Part model, mm, in its own coordinate system. Give positions to 0.01 mm unless a question says otherwise; leave off trailing zeros. Write each loop counter-clockwise with the first axis right and the second up, starting at its lowest first coordinate (ties: lowest second). Pieces come first, ordered by that corner, then holes. Notation, with made-up numbers: M 82,-10.75 L 125,-10.75 A12 ccw 125,11.25 Z; hole C -30,-39 d6. An arc over 180 degrees is marked long. Use a Markdown table: item, result.
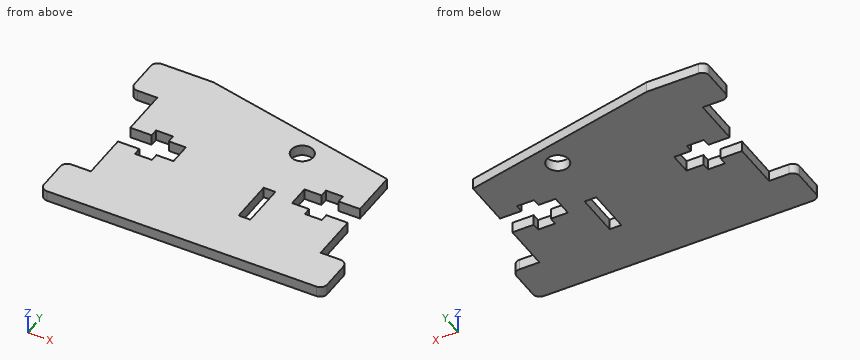
```python
from build123d import *

# Parameters (mm, degrees)
SKETCH_1_R      = 2.05
SKETCH_1_W      = 2.2
SKETCH_1_H      = 8.3
EXTRUDE_1_DEPTH = 2
FILLET_1_R      = 1.3


with BuildPart() as part:
    # 草图1 → 凸台-拉伸1 (new body)
    with BuildSketch(Plane.XY):
        Polygon((-35.523848217, 30.239854129), (-30.523848217, 30.239854129), (12.476151783, 30.239854129), (17.476151783, 30.239854129), (17.476151783, 38.239854129), (12.476151783, 38.239854129), (12.476151783, 47.189854129), (8.476151783, 47.189854129), (8.476151783, 45.739854129), (5.276151783, 45.739854129), (5.276151783, 47.189854129), (2.076151783, 47.189854129), (2.076151783, 51.289854129), (5.276151783, 51.289854129), (5.276151783, 52.739854129), (8.476151783, 52.739854129), (8.476151783, 51.289854129), (12.476151783, 51.289854129), (12.476151783, 60.239854129), (-24.523824953, 68.239854129), (-30.523848217, 68.239854129), (-35.523848217, 68.239854129), (-35.523848217, 60.239854129), (-30.523848217, 60.239854129), (-30.523848217, 51.289854129), (-26.523848217, 51.289854129), (-26.523848217, 52.739854129), (-23.323848217, 52.739854129), (-23.323848217, 51.289854129), (-20.123848217, 51.289854129), (-20.123848217, 47.189854129), (-23.323848217, 47.189854129), (-23.323848217, 45.739854129), (-26.523848217, 45.739854129), (-26.523848217, 47.189854129), (-30.523848217, 47.189854129), (-30.523848217, 38.239854129), (-35.523848217, 38.239854129), align=None)
        with Locations((-2.823848217, 59.239854129)):
            Circle(SKETCH_1_R, mode=Mode.SUBTRACT)
        with Locations((-2.823848217, 44.239854129)):
            Rectangle(SKETCH_1_W, SKETCH_1_H, mode=Mode.SUBTRACT)
    extrude(amount=EXTRUDE_1_DEPTH)

    # 圆角1
    fillet_1_edges = [part.edges().sort_by_distance(p)[0] for p in [
        (-35.523848217, 60.239854129, 1),
        (-35.523848217, 68.239854129, 1),
        (17.476151783, 38.239854129, 1),
        (17.476151783, 30.239854129, 1),
        (-35.523848217, 30.239854129, 1),
        (-35.523848217, 38.239854129, 1),
    ]]
    fillet(fillet_1_edges, radius=FILLET_1_R)


solid = part.part
```
1. Cut at A-A, the plane x = -31.5. Give the cut face in (y, z).
Findings below:
| item | result |
|---|---|
| outline | M 30.24,0 L 38.24,0 L 38.24,2 L 30.24,2 Z; M 60.24,0 L 68.24,0 L 68.24,2 L 60.24,2 Z |
2. Cut at B-B, the plane y = 58. Give the cut face in (x, z).
Findings below:
| item | result |
|---|---|
| outline | M -30.52,0 L -4.46,0 L -4.46,2 L -30.52,2 Z; M -1.19,0 L 12.48,0 L 12.48,2 L -1.19,2 Z |
3. Drop flat-ended pins along their axis: P1, Ø0.6, axis at y = 43, z = 0.5, coming from the -X side; P2, Ø1, axis at y = 38.5, z = 0.5, coming from the +X side; P3, Ø1, axis at x = -2.5, z = 0.5, coming from the +Y side; P4, Ø2, axis at x = 7, y = 45.5, coming from the -Z side. Give the stop position or say it passes through.
Findings below:
| item | result |
|---|---|
| P1 | x = -30.52 |
| P2 | x = 16.93 |
| P3 | y = 63.59 |
| P4 | z = 0 |
4. Drill centre lines: L1, parallel to X at y = 51.5, z = 0.45; L2, parallel to X at y = 46, z = 0.4; L3, parallel to X at y = 40.5, z = 0.3. Where is each one in solid material? Low to high.
Findings below:
| item | result |
|---|---|
| L1 | -30.52 to -26.52, -23.32 to 5.28, 8.48 to 12.48 |
| L2 | -30.52 to -26.52, -23.32 to -3.92, -1.72 to 5.28, 8.48 to 12.48 |
| L3 | -30.52 to -3.92, -1.72 to 12.48 |
5. Cut at D-D, the plane z = 1.5. State how many separate pieces and enclosed holes the cut face has, then the cut area to 3 significant figures.
Findings below:
| item | result |
|---|---|
| separate pieces | 1 |
| enclosed holes | 2 |
| area | 1,470 mm2 |
6. Cut at C-C, the plane x = -16. Give the cut face in (y, z).
Findings below:
| item | result |
|---|---|
| outline | M 30.24,0 L 66.4,0 L 66.4,2 L 30.24,2 Z |
